```python
from build123d import *

# Parameters (mm, degrees)
F1_DEPTH = 8
F2_W     = 30
F2_H     = 8
F3_DEPTH = 37
F6_D     = 15
F7_D     = 15
F7_DEPTH = 8


with BuildPart() as f1:
    # F0 (on Right) → F1 (new body)
    with BuildSketch(Plane.YZ):
        Polygon((-60, 45), (-90, 45), (-90, 0), (0, 0), (0, 45), (-30, 45), (-60, 25), align=None)
    extrude(amount=F1_DEPTH)

    # F2 (on face) → F3 (join)
    with BuildSketch(Plane.YZ.offset(8)):
        with Locations((-15, 4)):
            Rectangle(F2_W, F2_H)
        with Locations((-15, 41)):
            Rectangle(F2_W, F2_H)
    extrude(amount=F3_DEPTH)

    # F6 (through all)
    with Locations(Plane.XY.offset(45)):
        with Locations((22.5, -15)):
            Hole(F6_D / 2)

    # F7
    with Locations(Plane.YZ.offset(8)):
        with Locations((-75, 22.5)):
            Hole(F7_D / 2, depth=F7_DEPTH)


solid = f1.part
```
Work out the finished part from the listing and answer in its coordinate system (mm). A direction names the side the tool comes from. Give positions to 0.01 mm unless a question says otherwise; leave off trailing zeros. Write each loop counter-clockwise with the first axis right and the second up, starting at its lowest first coordinate (ties: lowest second). Pieces come first, ordered by that corner, then holes. Notation, with made-up numbers: (-8, -40) -> (42, -40) arc R16 ccw to (42, -14) -> close; hole circle Ø5 at (81.25, 53). An arc over 180 degrees is marked (long way). Write item = value, one per line.
Q1. Consider line 1 along Z through (x, y) = (2, -75); line 2 along Z through (x, y) = (11, -12.5); line 3 along Y through (x, z) = (22.5, 3). Determine where each line is inside the solid, lowest interval first.
Computed values:
line_1 = 0 to 15, 30 to 45
line_2 = 0 to 8, 37 to 45
line_3 = -30 to -22.5, -7.5 to 0
Q2. A tool of negligible diameter and unlimited length cuts with its end or side. For faces 4 (the flat face through (26, -30, 4)), 5 (the flat face through (4, -45, 35)), 6 (the flat face through (30.4, -15.2, 8)), from which of +Z, -Z, +X, -X, +Y, -Y can it reach the whole face along a straight path? Write none if from no direction.
Computed values:
face_4 = +Z, -Z, +X, -Y
face_5 = +Z, +X, -X
face_6 = +X, +Y, -Y
Q3. Section A-A on y = -15 is taken. Determine the outline of the cut face in (x, z), and give its area (3 significant figures).
Computed values:
outline = (0, 0) -> (15, 0) -> (15, 8) -> (8, 8) -> (8, 37) -> (15, 37) -> (15, 45) -> (0, 45) -> close; (30, 0) -> (45, 0) -> (45, 8) -> (30, 8) -> close; (30, 37) -> (45, 37) -> (45, 45) -> (30, 45) -> close
area = 712 mm^2
Q4. Section B-B on x = 22.5 is taken. Determine the outline of the cut face in (y, z), and give its area (3 significant figures).
Computed values:
outline = (-30, 0) -> (-22.5, 0) -> (-22.5, 8) -> (-30, 8) -> close; (-30, 37) -> (-22.5, 37) -> (-22.5, 45) -> (-30, 45) -> close; (-7.5, 0) -> (0, 0) -> (0, 8) -> (-7.5, 8) -> close; (-7.5, 37) -> (0, 37) -> (0, 45) -> (-7.5, 45) -> close
area = 240 mm^2
Q5. For a pull along X with two mould halves and no side action, classify faces 1 (the cylindrical face through (30, -15, 4)), 2 (the flat face through (26, -30, 41)), 3 (the flat face through (0, -46, 23)) as pulls with the +X half, pulls with the -X half, needs draft (parallel to the pull), parting line crosses it, or undercut.
Computed values:
face_1 = undercut
face_2 = needs draft
face_3 = pulls with the -X half
Q6. Flat-ended cylindrical pins translate along their axes: pin 1 Ø6.5 at (x, z) = (26, 42) entering from -Y; pin 2 Ø9 at (y, z) = (-75, 22.5) entering from -X; pin 3 Ø22.5 at (y, z) = (-46, 20.5) entering from +X. Find the tip coordinate at first contact, or state that the pin passes through.
Computed values:
pin_1 = -30
pin_2 = through
pin_3 = 8
Q7. Section C-C on y = -75 is taken. Determine the outline of the cut face in (x, z), and give its area (3 significant figures).
Computed values:
outline = (0, 0) -> (8, 0) -> (8, 15) -> (0, 15) -> close; (0, 30) -> (8, 30) -> (8, 45) -> (0, 45) -> close
area = 240 mm^2
Q8. Section D-D on z = 18 is taken. Determine the outline of the cut face in (x, y).
Computed values:
outline = (0, -90) -> (8, -90) -> (8, -81) -> (0, -81) -> close; (0, -69) -> (8, -69) -> (8, 0) -> (0, 0) -> close
